```python
from build123d import *

# Parameters (mm, degrees)
ESTRUSIONE_ESTRUSIONE1_DEPTH = 4
ESTRUSIONE_ESTRUSIONE2_DEPTH = 82
ESTRUSIONE_ESTRUSIONE3_START = 4
ESTRUSIONE_ESTRUSIONE3_DEPTH = 4
FORO_PER_VITE_M4_1_D         = 4.5
FORO_PER_VITE_M4_1_DEPTH     = 188
FORO_PER_VITE_M4_1_TIP       = 1.351936393
SCHIZZO6_R                   = 1.2
SCHIZZO6_W                   = 8.7
SCHIZZO6_H                   = 8.7
TAGLIO_ESTRUSIONE1_DEPTH     = 10
RACCORDO1_R                  = 10
RACCORDO2_R                  = 4


with BuildPart() as part:
    # Schizzo1 → Estrusione-Estrusione1 (new body)
    with BuildSketch(Plane.XY):
        with BuildLine():
            Line((-7, 0), (-7, 51.127312028))
            Line((-7, 51.127312028), (-39.227701012, 89.53479049))
            Line((-39.227701012, 89.53479049), (-31.567256581, 95.962666587))
            Line((-31.567256581, 95.962666587), (7, 50))
            Line((7, 50), (7, 0))
            ThreePointArc((7, 0), (0, 7), (-7, 0))
        make_face()
    extrude(amount=ESTRUSIONE_ESTRUSIONE1_DEPTH)

    # Schizzo4 → Estrusione-Estrusione2 (add)
    with BuildSketch(Plane.XY):
        Polygon((-39.227701012, 89.53479049), (-23.15801077, 70.383679412), (-20.859877441, 72.312042241), (-36.929567683, 91.463153319), align=None)
    extrude(amount=-ESTRUSIONE_ESTRUSIONE2_DEPTH)

    # Schizzo5 → Estrusione-Estrusione3 (add)
    with BuildSketch(Plane(origin=(0, 0, -82), x_dir=(-1, 0, 0), z_dir=(0, 0, -1)).offset(ESTRUSIONE_ESTRUSIONE3_START)):
        with BuildLine():
            Line((-7, 0), (-7, 50))
            Line((-7, 50), (31.567256581, 95.962666587))
            Line((31.567256581, 95.962666587), (39.227701012, 89.53479049))
            Line((39.227701012, 89.53479049), (7, 51.127312028))
            Line((7, 51.127312028), (7, 0))
            ThreePointArc((7, 0), (0, 7), (-7, 0))
        make_face()
    extrude(amount=-ESTRUSIONE_ESTRUSIONE3_DEPTH)

    # Foro per Vite M4-1
    with Locations(Plane.XY.offset(4)):
        with Locations((0, 12)):
            Hole(FORO_PER_VITE_M4_1_D / 2, depth=FORO_PER_VITE_M4_1_DEPTH)
            with Locations((0, 0, -(FORO_PER_VITE_M4_1_DEPTH + FORO_PER_VITE_M4_1_TIP / 2))):  # 118° drill point
                Cone(0, FORO_PER_VITE_M4_1_D / 2, FORO_PER_VITE_M4_1_TIP, mode=Mode.SUBTRACT)

    # Schizzo6 → Taglio-Estrusione1 (cut)
    with BuildSketch(Plane(origin=(23.365651345, 19.606109426, 0), x_dir=(0, 0, -1), z_dir=(0.7660444431189758, 0.642787609686542, 0))):
        with Locations(Location((30.05, 91.452708888, 0), (0, 0, 90))):
            Circle(SCHIZZO6_R)
        with Locations(Location((41.65, 91.452708888, 0), (0, 0, 90))):
            Circle(SCHIZZO6_R)
        with Locations(Location((30.05, 71.152708888, 0), (0, 0, 90))):
            Circle(SCHIZZO6_R)
        with Locations(Location((41.65, 71.152708888, 0), (0, 0, 90))):
            Circle(SCHIZZO6_R)
        with Locations((41, 81.502708888)):
            Rectangle(SCHIZZO6_W, SCHIZZO6_H)
    extrude(amount=-TAGLIO_ESTRUSIONE1_DEPTH, mode=Mode.SUBTRACT)

    # Raccordo1
    raccordo1_edges = [part.edges().sort_by_distance(p)[0] for p in [
        (-7, 51.127312028, 2),
        (7, 50, 2),
        (-7, 51.127312028, -84),
        (7, 50, -84),
    ]]
    fillet(raccordo1_edges, radius=RACCORDO1_R)

    # Raccordo2
    raccordo2_edges = [part.edges().sort_by_distance(p)[0] for p in [
        (-22.008944106, 71.347860827, -82),
        (-22.008944106, 71.347860827, 0),
    ]]
    fillet(raccordo2_edges, radius=RACCORDO2_R)


solid = part.part
```
Input: part model. Units: mm. Frame: model coordinates. A direction names the side the tool comes from. Round coordinates to 2 decimals unless told otherwise and drop trailing zeros. Loops run counter-clockwise (first coordinate to the right, second up) from the corner with the lowest first, then second, coordinate; pieces in that order, holes last. Notation, with made-up numbers: (28.25, -23.5) - (47.25, -23.5) arc R34 ccw to (47.25, 6.5) - close; hole circle Ø6 at (-6.75, 22). An arc over 180 degrees is marked (long way). One line per item, written item: value. Start each with the question number.
(1) Contact query for flat-ended pins moving along their axis: P1, Ø12, axis at x = -16, z = -56, coming from the -Y side; P2, Ø3, axis at y = 30.5, z = 1.5, coming from the -X side; P3, Ø4, axis at x = -21.5, z = -39, coming from the -Y side. Output: stop coordinate, or through.
(2) Section A-A, the plane y = 41. Return loops of the section in (x, z), plus the area to 3 significant figures.
(3) Ray query, line 1 (Z direction, x = -4.5, y = 41); line 2 (Y direction, x = 0, z = 1); line 3 (X direction, y = 73.5, z = -4.5). Return the intervals inside material, ascending. Write a range as [from, to].
(4) Section D-D, the plane x = -17. Return loops of the section in (y, z).
(5) Section B-B, the plane y = 12. Return loops of the section in (x, z), plus the area to 3 significant figures.
(6) Draft query along X for faces 5 (the cylindrical face through (0.29, 14.23, 1.97)), 6 (the flat face through (-30, 81, -45.35)), 7 (the flat face through (-22.03, 71.33, -40.48)). Return one class per face: +X half, -X half, draft (parallel to the pull), parting line (faces both ways), or undercut.
(7) Section C-C, the plane x = 0. Return loops of the section in (y, z).
(8) Access query for faces 1 (the flat face through (-27.36, 77.76, -40.94)), 2 (the cylindrical face through (0, 7, -84)), 3 (the cylindrical face through (-21.26, 70.488, -1.203)), 4 (the flat face through (-25.407, 77.732, -40.426)). Directions: +Z, -Z, +X, -X, +Y, -Y. A direction counts if a zero-diameter tool reaches every point of the face in a straight line with its end or side. Return the directions, or none.
Results below:
1. P1: y = 71.36
1. P2: x = -7
1. P3: y = 70.38
2. outline: (-7, -86) - (7, -86) - (7, -82) - (-7, -82) - close; (-7, 0) - (7, 0) - (7, 4) - (-7, 4) - close
2. area: 112 mm^2
3. line 1: [-86, -82], [0, 4]
3. line 2: [7, 9.75], [14.25, 58.34]
3. line 3: [-25.77, -21.86]
4. outline: (63.04, -86) - (78.6, -86) - (78.6, -82) - (63.04, -82) - close; (63.04, 0) - (78.6, 0) - (78.6, 4) - (63.04, 4) - close
5. outline: (-7, -86) - (-2.25, -86) - (-2.25, -82) - (-7, -82) - close; (-7, 0) - (-2.25, 0) - (-2.25, 4) - (-7, 4) - close; (2.25, -86) - (7, -86) - (7, -82) - (2.25, -82) - close; (2.25, 0) - (7, 0) - (7, 4) - (2.25, 4) - close
5. area: 76.0 mm^2
6. face 5: undercut
6. face 6: draft
6. face 7: +X half
7. outline: (7, -86) - (9.75, -86) - (9.75, -82) - (7, -82) - close; (7, 0) - (9.75, 0) - (9.75, 4) - (7, 4) - close; (14.25, -86) - (58.34, -86) - (58.34, -82) - (14.25, -82) - close; (14.25, 0) - (58.34, 0) - (58.34, 4) - (14.25, 4) - close
8. face 1: -X, +Y
8. face 2: +Z, -Z, -Y
8. face 3: +X, -Y
8. face 4: +X, +Y
